from build123d import *

# Parameters (mm, degrees)
SKETCH1_W           = 240
SKETCH1_H           = 45
BOSS_EXTRUDE1_DEPTH = 34.9
FILLET1_R           = 23
CUT_EXTRUDE1_START  = -7.5
SKETCH2_W           = 49.564850137
SKETCH2_H           = 45.01227926
CUT_EXTRUDE1_DEPTH  = 19.9
SKETCH3_R           = 6
CUT_EXTRUDE2_DEPTH  = 154.260575491
SKETCH4_R           = 6.5
CUT_EXTRUDE3_DEPTH  = 154.260575491
SCALE1_SCALE        = 0.31


with BuildPart() as part:
    # Sketch1 → Boss-Extrude1 (new body)
    with BuildSketch(Plane(origin=(0, 0, 0), x_dir=(1, 0, 0), z_dir=(0, 1, 0))):
        with Locations((24.613815765, -14.36746988)):
            Rectangle(SKETCH1_W, SKETCH1_H)
    extrude(amount=BOSS_EXTRUDE1_DEPTH)

    # Fillet1
    # the kernel refuses this fillet: 23 mm, written as the material it takes off along each edge
    with BuildSketch(Plane(origin=(-95.386184235, -57.5, 36.86746988), x_dir=(1, 0, 0), z_dir=(0, 1, 0))) as fillet1_piece_1:
        with BuildLine():
            CenterArc((FILLET1_R, FILLET1_R), FILLET1_R, 180, 90)
            Line((0, FILLET1_R), (0, 0))
            Line((0, 0), (FILLET1_R, 0))
        make_face()
    extrude(amount=149.9, mode=Mode.SUBTRACT)
    with BuildSketch(Plane(origin=(-95.386184235, -57.5, -8.13253012), x_dir=(1, 0, 0), z_dir=(0, 1, 0)), Plane(origin=(144.613815765, -57.5, 36.86746988), x_dir=(-1, 0, 0), z_dir=(0, 1, 0)), Plane(origin=(144.613815765, -57.5, -8.13253012), x_dir=(0, 0, 1), z_dir=(0, 1, 0))) as fillet1_piece_2:
        with BuildLine():
            CenterArc((FILLET1_R, -FILLET1_R), FILLET1_R, 90, 90)
            Line((0, -FILLET1_R), (0, 0))
            Line((0, 0), (FILLET1_R, 0))
        make_face()
    extrude(amount=149.9, mode=Mode.SUBTRACT)

    # Sketch2 → Cut-Extrude1 (cut)
    with BuildSketch(Plane(origin=(0, 34.9, 0), x_dir=(1, 0, 0), z_dir=(0, 1, 0)).offset(CUT_EXTRUDE1_START)):
        with Locations((129.390805409, -14.37360951)):
            Rectangle(SKETCH2_W, SKETCH2_H)
    extrude(amount=-CUT_EXTRUDE1_DEPTH, mode=Mode.SUBTRACT)

    # Sketch3 → Cut-Extrude2 (cut, through all)
    with BuildSketch(Plane.XZ):
        with Locations(Location((124.60838034, 14.935006331, 0), (0, 0, 270))):
            Circle(SKETCH3_R)
    extrude(amount=-CUT_EXTRUDE2_DEPTH, mode=Mode.SUBTRACT)

    # Sketch4 → Cut-Extrude3 (cut, through all)
    with BuildSketch(Plane.XZ):
        with Locations(Location((-56.380748811, 14.36746988, 0), (0, 0, 270))):
            Circle(SKETCH4_R)
    extrude(amount=-CUT_EXTRUDE3_DEPTH, mode=Mode.SUBTRACT)


with BuildPart() as part_1:
    # Scale1: scaled about (0, 0, 0)
    add(part.part.scale(SCALE1_SCALE))


solid = part_1.part
Geometry: final body of the model. Coordinates: model frame, mm. A direction names the side the tool comes from. Round coordinates to 2 decimals unless told otherwise and drop trailing zeros. Loops run counter-clockwise (first coordinate to the right, second up) from the corner with the lowest first, then second, coordinate; pieces in that order, holes last. Notation, with made-up numbers: M 8,50 L 54,50 A9 cw 54,55 Z; hole C 7,55 d11. An arc over 180 degrees is marked long. Put each result on its own line as item: value. Start each with the question number.
(1) Section query C-C (y = 6.25). Return loops of the section in (x, z) (3 decimals).
(2) Contact query for flat-ended pins moving along their axis: pin 1 Ø2 at (y, z) = (5, 9) entering from -X; pin 2 Ø5 at (y, z) = (5, 8) entering from +X; pin 3 Ø3.5 at (x, z) = (-17.48, 4.45) entering from -Y. Output: stop coordinate, or through.
(3) Section query A-A (x = 33.5). Return loops of the section in (y, z) (3 decimals).
(4) Section query D-D (y = 9.5). Return loops of the section in (x, z) (3 decimals), then the cut area to 3 significant figures.
(5) Section query B-B (z = 5.25). Return loops of the section in (x, y) (3 decimals).
(6) Draft query along X for faces 3 (the face through (42.742, 1.146, -0.433)), 4 (the face through (-27.37, 5.33, -0.54)), 5 (the face through (40.473, 9.64, 4.872)), 6 (the face through (7, 10.819, 4)). Return one class per face: +X half, -X half, draft (parallel to the pull), parting line (faces both ways), or undercut.
(7) Material intervals for line 1 along Y through (x, z) = (41, 2) (3 decimals); line 2 along X through (y, z) = (5, 4.5); line 3 along Z through (x, y) = (38.5, 9.5), sorted ascending. Write a range as [from, to].
(8) Set-up query: faces 1 (the face through (32.429, 5, 5)), 2 (the face through (7, 5, 11.429)). Return all of +Z, -Z, +X, -X, +Y, -Y with unobstructed straight access to the full face (end or side cutting, diameter ignored); none if empty.
Findings below:
1. outline: M -29.568,4.454 A7.13 ccw -22.44,-2.521 L 32.429,-2.521 L 32.429,11.429 L -22.44,11.429 A7.13 ccw Z; hole C -17.478,4.454 d4.03
2. pin 1: stops at x = -28.53
2. pin 2: stops at x = 32.43
2. pin 3: passes through
3. outline: M 0,-2.521 L 2.325,-2.521 L 2.325,11.429 L 0,11.429 Z; M 8.494,-2.521 L 10.819,-2.521 L 10.819,11.429 L 8.494,11.429 Z
4. outline: M -29.568,4.454 A7.13 ccw -22.44,-2.521 L 37.7,-2.521 A7.13 ccw 44.829,4.454 A7.13 ccw 37.7,11.429 L -22.44,11.429 A7.13 ccw Z; hole C -17.478,4.454 d4.03; hole C 38.629,4.63 d3.72
4. area: 971 mm2
5. outline: M -29.506,0 L -19.329,0 L -19.329,10.819 L -29.506,10.819 Z; M -15.627,0 L 36.875,0 L 36.875,2.325 L 32.429,2.325 L 32.429,8.494 L 36.875,8.494 L 36.875,10.819 L -15.627,10.819 Z; M 40.382,0 L 44.767,0 L 44.767,2.325 L 40.382,2.325 Z; M 40.382,8.494 L 44.767,8.494 L 44.767,10.819 L 40.382,10.819 Z
6. face 3: +X half
6. face 4: -X half
6. face 5: undercut
6. face 6: draft
7. line 1: y = [0, 2.325], [8.494, 10.819]
7. line 2: x = [-29.57, -19.49], [-15.46, 32.43]
7. line 3: z = [-2.48, 2.77], [6.49, 11.38]
8. face 1: +Z, -Z, +X
8. face 2: +Z, +X, -X, +Y, -Y
